Source: three-view drawing plus pictorial views. Frame: mm from the lowest corner of the part. Coordinates: 2 decimals unless noted, no trailing zeros. Write each loop counter-clockwise with the first axis right and the second up, starting at its lowest first coordinate (ties: lowest second). Pieces come first, ordered by that corner, then holes. Notation, with made-up numbers: (38.25, 9) - (65.25, 9) arc R34 cw to (65.25, 40) - close; hole circle Ø7 at (78, -15.5). An arc over 180 degrees is marked (long way). Put each result on its own line as item: value. Start each with the question number.
1. Pin query (flat end, axial travel): pin 1 (3 mm diameter, centred on x = 58, y = 15.5, fed in from +Z); pin 2 (3.5 mm diameter, centred on x = 50.8, z = 50.8, fed in from -Y); pin 3 (8 mm diameter, centred on x = 60.5, y = 15, fed in from -Z); pin 4 (2 mm diameter, centred on y = 17, z = 46.5, fed in from -X). Return the tip coordinate at first contact, or that it passes through.
2. Cut plane C-C, the plane x = 74. Return loops of the section in (y, z) (3 decimals), and give its area (3 significant figures).
3. Cut plane D-D, the plane y = 17.25. Return loops of the section in (x, z) (1 decimal), and give its area (3 significant figures).
4. Line query: line 1 (Y direction, x = 68.5, z = 97) (3 decimals); line 2 (Z direction, x = 50.8, y = 7.5); line 3 (Z direction, x = 50.8, y = 10) (1 decimal). Output: solid intervals per line, ascending.
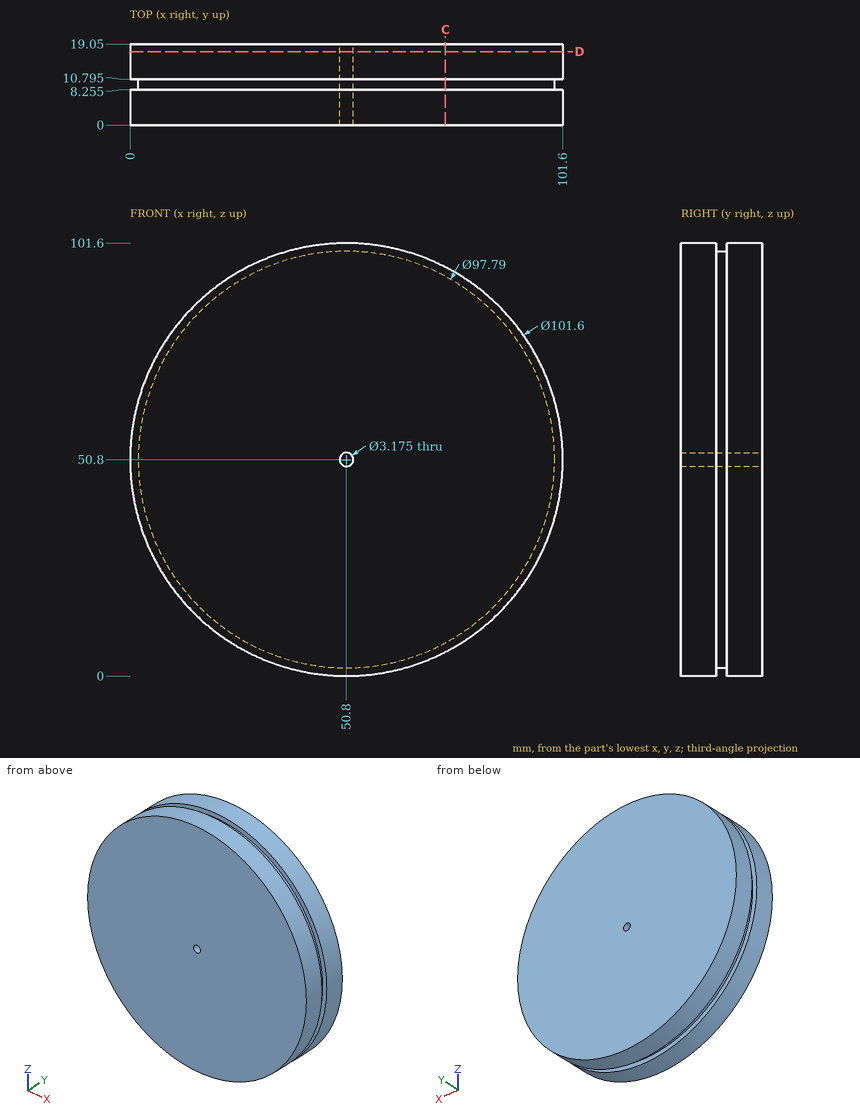
Report:
1. pin 1: stops at z = 101.28
1. pin 2: stops at y = 0
1. pin 3: stops at z = 0.32
1. pin 4: stops at x = 0.11
2. outline: (0, 5.607) - (8.255, 5.607) - (8.255, 7.76) - (10.795, 7.76) - (10.795, 5.607) - (19.05, 5.607) - (19.05, 95.993) - (10.795, 95.993) - (10.795, 93.84) - (8.255, 93.84) - (8.255, 95.993) - (0, 95.993) - close
2. area: 1,710 mm^2
3. outline: circle Ø101.6 at (50.8, 50.8); hole circle Ø3.2 at (50.8, 50.8)
3. area: 8,100 mm^2
4. line 1: y = 0 to 8.255, 10.795 to 19.05
4. line 2: z = 0 to 49.21, 52.39 to 101.6
4. line 3: z = 1.9 to 49.2, 52.4 to 99.7
